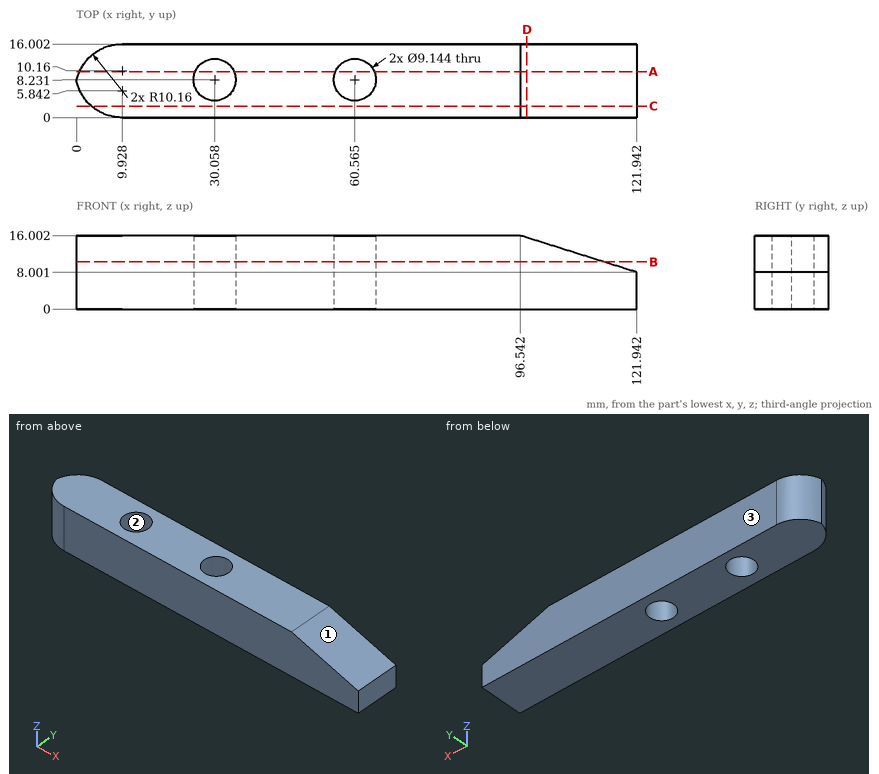
Study the drawing (mm; zero at the part's minimum x, y, z) and answer. Coordinates: 2 decimals unless noted, no trailing zeros. Write each loop counter-clockwise with the first axis right and the second up, starting at its lowest first coordinate (ties: lowest second). Pieces come first, ordered by that corner, then holes. Notation, with made-up numbers: M 28.25,15 L 49.25,15 A34 ccw 49.25,48 Z; hole C 1.25,-33.5 d6. An arc over 180 degrees is marked long. Use a Markdown table: item, result. Add a question column.
1. Section C-C (y = 2.5) is taken. Give the vertices of the cut face in (x, z).
2. Section D-D (x = 98) is taken. Give the vertices of the cut face in (y, z).
3. Straight lines are drawn through the part: line 1 along X through (y, z) = (11.25, 3) (1 decimal); line 2 along X through (y, z) = (4.5, 1.5) (1 decimal); line 3 along Y through (x, z) = (33, 15). For each, find the intervals that lie inside material, in ascending order. Write a range as [from, to].
4. For a pull along X with two mould halves and no side action, classify the marked faces 1, 2 and 3 as +X half, -X half, draft (parallel to the pull), parting line (faces both ways), or undercut.
5. Section B-B (z = 10.25) is taken. Give the vertices of the cut face in (x, y) (1 decimal).
6. Given P1, Ø8, axis at x = 60.57, y = 8.23, coming from the -Z side, flat-ended and moving along its own axis, determine where the tip first touches the part or whether it passes through.
7. Section A-A (y = 10) is taken. Give the vertices of the cut face in (x, z).
Data:
| question | item | result |
|---|---|---|
| 1 | outline | M 3.25,0 L 121.94,0 L 121.94,8 L 96.54,16 L 3.25,16 Z |
| 2 | outline | M 0,0 L 16,0 L 16,15.54 L 0,15.54 Z |
| 3 | line 1 | x = [1.3, 26.6], [33.5, 57.1], [64, 121.9] |
| 3 | line 2 | x = [1.5, 27.4], [32.7, 57.9], [63.2, 121.9] |
| 3 | line 3 | y = [0, 4.73], [11.73, 16] |
| 4 | face 1 | +X half |
| 4 | face 2 | undercut |
| 4 | face 3 | draft |
| 5 | outline | M 0,8 A10.2 ccw 9.9,0 L 114.8,0 L 114.8,16 L 9.9,16 A10.2 ccw Z; hole C 30.1,8.2 d9.1; hole C 60.6,8.2 d9.1 |
| 6 | P1 | passes through |
| 7 | outline | M 0.66,0 L 25.84,0 L 25.84,16 L 0.66,16 Z; M 34.27,0 L 56.35,0 L 56.35,16 L 34.27,16 Z; M 64.78,0 L 121.94,0 L 121.94,8 L 96.54,16 L 64.78,16 Z |
